from build123d import *

# Parameters (mm, degrees)
BOSS_EXTRUDE2_DEPTH = 20
SKETCH2_W           = 2
SKETCH2_H           = 9.242730417
CUT_EXTRUDE1_DEPTH  = 20
SKETCH3_W           = 1.5
SKETCH3_H           = 5.716408543
BOSS_EXTRUDE3_DEPTH = 20
SKETCH4_R           = 1
CUT_EXTRUDE2_DEPTH  = 11.65
FILLET1_R           = 4


with BuildPart() as part:
    # Sketch1 → Boss-Extrude2 (new body)
    with BuildSketch(Plane(origin=(0, 0, 0), x_dir=(0, 0, -1), z_dir=(1, 0, 0))):
        with BuildLine():
            Line((8.15, 11.4), (8.15, 0))
            ThreePointArc((8.15, 0), (0, -8.15), (-8.15, 0))
            Line((-8.15, 0), (-8.15, 11.4))
            ThreePointArc((-8.15, 11.4), (0, 19.55), (8.15, 11.4))
        make_face()
        with BuildLine():
            ThreePointArc((2.904067302, 7.391397612), (0, 16.35), (-2.904067302, 7.391397612))
            ThreePointArc((-2.904067302, 7.391397612), (-2.493172041, 6.511986737), (-3.022190844, 5.698145532))
            ThreePointArc((-3.022190844, 5.698145532), (0, -6.45), (3.022190844, 5.698145532))
            ThreePointArc((3.022190844, 5.698145532), (2.493172041, 6.511986737), (2.904067302, 7.391397612))
        make_face(mode=Mode.SUBTRACT)
    extrude(amount=BOSS_EXTRUDE2_DEPTH)

    # Sketch2 → Cut-Extrude1 (cut)
    with BuildSketch(Plane(origin=(20, 0, 0), x_dir=(0, 0, -1), z_dir=(1, 0, 0))):
        with Locations((0, -7.363862564)):
            Rectangle(SKETCH2_W, SKETCH2_H)
    extrude(amount=-CUT_EXTRUDE1_DEPTH, mode=Mode.SUBTRACT)

    # Sketch3 → Boss-Extrude3 (add)
    with BuildSketch(Plane(origin=(20, 0, 0), x_dir=(0, 0, -1), z_dir=(1, 0, 0))):
        with Locations((-1.75, -9.230213374)):
            Rectangle(SKETCH3_W, SKETCH3_H)
        with Locations((1.75, -9.230213374)):
            Rectangle(SKETCH3_W, SKETCH3_H)
    extrude(amount=-BOSS_EXTRUDE3_DEPTH)

    # Sketch4 → Cut-Extrude2 (cut, through all)
    with BuildSketch(Plane(origin=(0, 0, -2.5), x_dir=(-1, 0, 0), z_dir=(0, 0, -1))):
        with Locations((-14, -10.088417645)):
            Circle(SKETCH4_R)
        with Locations((-6, -10.088417645)):
            Circle(SKETCH4_R)
    extrude(amount=-CUT_EXTRUDE2_DEPTH, mode=Mode.SUBTRACT)

    # Fillet1
    fillet1_edges = [part.edges().sort_by_distance(p)[0] for p in [
        (20, -12.088417645, 1.75),
        (0, -12.088417645, 1.75),
        (20, -12.088417645, -1.75),
        (0, -12.088417645, -1.75),
    ]]
    fillet(fillet1_edges, radius=FILLET1_R)


solid = part.part
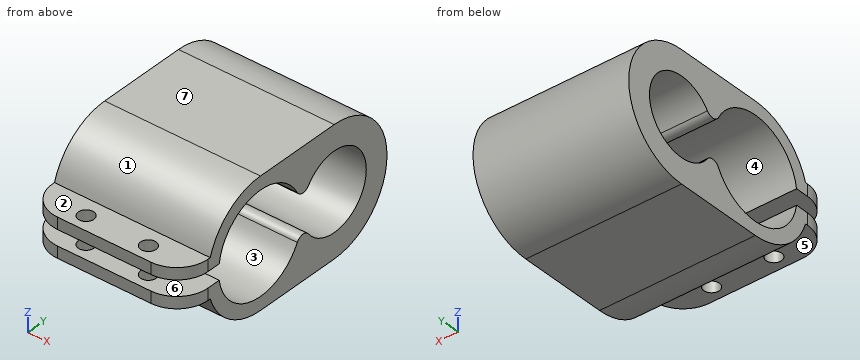
Design review of the part built by this model. Coordinates are the model's own, in mm. Face numbers are marked on the shaded views. A direction names the side the tool comes from. Round coordinates to 2 decimals unless told otherwise and drop trailing zeros. Loops run counter-clockwise (first coordinate to the right, second up) from the corner with the lowest first, then second, coordinate; pieces in that order, holes last. Notation, with made-up numbers: (-25.5, 48) -> (16.5, 48) arc R24 cw to (16.5, 60) -> close; hole circle Ø4 at (80, -5.5). An arc over 180 degrees is marked (long way). Use one line per item in the form item = value. Start each with the question number.
Q1. Wall thickness on line 1 along Z through (x, y) = (16.75, -10); line 2 along Z through (x, y) = (6, 6.5); line 3 along Y through (x, z) = (5, 2.75): over which ranges is each line inside the solid? List them lowest first. Write a range as [from, to].
Q2. We need section B-B on x = 14. Give the boundary of the cut face in (y, z).
Q3. Draft analysis for pull direction Y (two halves, no side actions). For the marked faces 1, 2 and 3, state which applies: +Y half, -Y half, draft (parallel to the pull), parting line (faces both ways), or undercut.
Q4. For pin 1 Ø8 at (y, z) = (11.4, 0) entering from +X; pin 2 Ø2.5 at (x, y) = (6, -10.09) entering from +Z; pin 3 Ø3 at (x, y) = (5, -9) entering from -Z; pin 4 Ø3.5 at (x, y) = (10.5, -9) entering from -Z, all flat-tipped, find the tip position at first contact; note any pin that passes through.
Q5. We need section A-A on z = -2. Give the boundary of the cut face in (x, y), then the cut area to 3 significant figures.
Q6. Machinability: for the marked faces 4, 5, 6 and 7, which of the approach directions +Z, -Z, +X, -X, +Y, -Y give a long, thin tool a straight path to every point of the face, cutting with its end or side? Answer none if there is none.
Q7. We need section C-C on y = 4.5. Give the boundary of the cut face in (x, z), then the cut area to 3 significant figures.
Q8. We need section D-D on z = 5.75. Give the boundary of the cut face in (x, y), then the cut area to 3 significant figures.
Calculated:
q1.line_1 = [-2.5, -1], [1, 2.5]
q1.line_2 = [-8.15, -2.49], [2.49, 8.15]
q1.line_3 = [-7.67, -5.83], [5.91, 7.25], [15.52, 19.07]
q2.outline = (-12.09, -2.5) -> (-11.09, -2.5) -> (-11.09, -1) -> (-12.09, -1) -> close; (-12.09, 1) -> (-11.09, 1) -> (-11.09, 2.5) -> (-12.09, 2.5) -> close; (-9.09, -2.5) -> (-7.76, -2.5) arc R8.15 ccw to (0, -8.15) -> (11.4, -8.15) arc R8.15 ccw to (11.4, 8.15) -> (0, 8.15) arc R8.15 ccw to (-7.76, 2.5) -> (-9.09, 2.5) -> (-9.09, 1) -> (-6.37, 1) arc R6.45 cw to (5.7, 3.02) arc R1 ccw to (7.39, 2.9) arc R4.95 cw (long way) to (7.39, -2.9) arc R1 ccw to (5.7, -3.02) arc R6.45 cw to (-6.37, -1) -> (-9.09, -1) -> close
q3.face_1 = -Y half
q3.face_2 = draft
q3.face_3 = undercut
q4.pin_1 = through
q4.pin_2 = 2.5
q4.pin_3 = -3.19
q4.pin_4 = -3.72
q5.outline = (0, -8.09) arc R4 ccw to (4, -12.09) -> (16, -12.09) arc R4 ccw to (20, -8.09) -> (20, -6.13) -> (0, -6.13) -> close; (0, 15.93) -> (20, 15.93) -> (20, 19.3) -> (0, 19.3) -> close; hole circle Ø2 at (6, -10.09); hole circle Ø2 at (14, -10.09)
q5.area = 173 mm²
q6.face_4 = +X, -X
q6.face_5 = -Z, +X, -X, -Y
q6.face_6 = +X, -X, -Y
q6.face_7 = +Z, +X, -X, +Y, -Y
q7.outline = (0, -8.15) -> (20, -8.15) -> (20, -4.62) -> (0, -4.62) -> close; (0, 4.62) -> (20, 4.62) -> (20, 8.15) -> (0, 8.15) -> close
q7.area = 141 mm²
q8.outline = (0, -5.78) -> (20, -5.78) -> (20, -2.92) -> (0, -2.92) -> close; (0, 2.92) -> (20, 2.92) -> (20, 17.18) -> (0, 17.18) -> close
q8.area = 342 mm²
